```python
from build123d import *

# Parameters (mm, degrees)
SKETCH1_W           = 150
SKETCH1_H           = 60
BOSS_EXTRUDE1_DEPTH = 20
SKETCH2_W           = 22
SKETCH2_H           = 60
BOSS_EXTRUDE2_DEPTH = 10
SKETCH3_W           = 26.3
SKETCH3_H           = 26.3
CUT_EXTRUDE1_DEPTH  = 84.216584885
SKETCH4_R           = 2.2
CUT_EXTRUDE2_DEPTH  = 101.623058987
SKETCH5_R           = 2.8
CUT_EXTRUDE3_DEPTH  = 6
SKETCH6_R           = 4
CUT_EXTRUDE4_DEPTH  = 2


with BuildPart() as part:
    # Sketch1 → Boss-Extrude1 (new body)
    with BuildSketch(Plane(origin=(0, 0, 0), x_dir=(1, 0, 0), z_dir=(0, 1, 0))):
        Rectangle(SKETCH1_W, SKETCH1_H)
    extrude(amount=BOSS_EXTRUDE1_DEPTH)

    # Sketch2 → Boss-Extrude2 (add)
    with BuildSketch(Plane(origin=(0, 20, 0), x_dir=(1, 0, 0), z_dir=(0, 1, 0))):
        with Locations((-64, 0)):
            Rectangle(SKETCH2_W, SKETCH2_H)
    extrude(amount=BOSS_EXTRUDE2_DEPTH)

    # Sketch3 → Cut-Extrude1 (cut, through all)
    with BuildSketch(Plane(origin=(0, 20, 0), x_dir=(1, 0, 0), z_dir=(0, 1, 0))):
        with Locations((-22.5, 0)):
            Rectangle(SKETCH3_W, SKETCH3_H)
    extrude(amount=-CUT_EXTRUDE1_DEPTH, mode=Mode.SUBTRACT)

    # Sketch4 → Cut-Extrude2 (cut, through all)
    with BuildSketch(Plane.XY.offset(30)):
        with Locations((-22.5, 10)):
            Circle(SKETCH4_R)
    extrude(amount=-CUT_EXTRUDE2_DEPTH, mode=Mode.SUBTRACT)

    # Sketch5 → Cut-Extrude3 (cut)
    with BuildSketch(Plane.XY.offset(30)):
        with Locations((-22.5, 10)):
            Circle(SKETCH5_R)
    extrude(amount=-CUT_EXTRUDE3_DEPTH, mode=Mode.SUBTRACT)

    # Sketch6 → Cut-Extrude4 (cut)
    with BuildSketch(Plane(origin=(0, 0, 0), x_dir=(-1, 0, 0), z_dir=(0, -1, 0))):
        with Locations(Location((0, 0, 0), (0, 0, 90))):
            Circle(SKETCH6_R)
        with Locations(Location((-55, 0, 0), (0, 0, 90))):
            Circle(SKETCH6_R)
        with Locations(Location((55, 0, 0), (0, 0, 90))):
            Circle(SKETCH6_R)
    extrude(amount=-CUT_EXTRUDE4_DEPTH, mode=Mode.SUBTRACT)


solid = part.part
```
Check sheet for the modelled part. Datum: model origin and axes. Units: mm. A direction names the side the tool comes from. Round coordinates to 2 decimals unless told otherwise and drop trailing zeros. Loops run counter-clockwise (first coordinate to the right, second up) from the corner with the lowest first, then second, coordinate; pieces in that order, holes last. Notation, with made-up numbers: (-34, -37) - (-15, -37) arc R30 ccw to (-15, -9) - close; hole circle Ø11 at (79, 34). An arc over 180 degrees is marked (long way). Write item = value, one per line. Start each with the question number.
Q1. Section check A-A (x = -22.5). Record the boundary of the cut face in (y, z).
Q2. Section check D-D (y = 10). Record the boundary of the cut face in (x, z).
Q3. Section check C-C (z = 0). Record the boundary of the cut face in (x, y), plus the area to 3 significant figures.
Q4. Access from +Z, -Z, +X, -X, +Y, -Y to the whole of each face (thin tool, end or side, straight path). Record for faces 4 (the face through (-25.3, 10.1, 27)), 5 (the face through (-53, 25, 0)), 6 (the face through (55, 2, 0)), 7 (the face through (-22.7, 12.4, -13.15)), 8 (the face through (-20.4, 10.66, 18.65)).
Q5. Thickness scan on L1, parallel to X at y = 1.25, z = 0; L2, parallel to Y at x = 56, z = 25.5; L3, parallel to Z at x = -30.5, y = 1.75. Record the ranges inside material, lowest first.
Q6. Section check B-B (y = 17.25). Record the boundary of the cut face in (x, z).
Q7. Release check for a two-part mould opening along Y. For faces 1 (the face through (-64, 30, 0)), 2 (the face through (-1, 11, 30)), 3 (the face through (-21, 8, 24)) record: pulls with the +Y half, pulls with the -Y half, needs draft (parallel to the pull), parting line crosses it, or undercut.
Q8. Depth check by flat-ended pin: P1, Ø3.5, axis at x = -22.5, y = 10, coming from the -Z side; P2, Ø10.5, axis at x = 55, z = 0, coming from the +Y side; P3, Ø9, axis at x = -55.5, z = 1.5, coming from the -Y side; P4, Ø5, axis at y = 25.5, z = -5, coming from the +X side. Enter the tip coordinate at first touch or a pass-through.
Derived:
q1.outline = (0, -30) - (7.8, -30) - (7.8, -13.15) - (0, -13.15) - close; (0, 13.15) - (7.8, 13.15) - (7.8, 24) - (7.2, 24) - (7.2, 30) - (0, 30) - close; (12.2, -30) - (20, -30) - (20, -13.15) - (12.2, -13.15) - close; (12.2, 13.15) - (20, 13.15) - (20, 30) - (12.8, 30) - (12.8, 24) - (12.2, 24) - close
q2.outline = (-75, -30) - (-24.7, -30) - (-24.7, -13.15) - (-35.65, -13.15) - (-35.65, 13.15) - (-24.7, 13.15) - (-24.7, 24) - (-25.3, 24) - (-25.3, 30) - (-75, 30) - close; (-20.3, -30) - (75, -30) - (75, 30) - (-19.7, 30) - (-19.7, 24) - (-20.3, 24) - (-20.3, 13.15) - (-9.35, 13.15) - (-9.35, -13.15) - (-20.3, -13.15) - close
q3.outline = (-75, 0) - (-59, 0) - (-59, 2) - (-51, 2) - (-51, 0) - (-35.65, 0) - (-35.65, 20) - (-53, 20) - (-53, 30) - (-75, 30) - close; (-9.35, 0) - (-4, 0) - (-4, 2) - (4, 2) - (4, 0) - (51, 0) - (51, 2) - (59, 2) - (59, 0) - (75, 0) - (75, 20) - (-9.35, 20) - close
q3.area = 2,650 mm^2
q4.face_4 = +Z
q4.face_5 = +Z, -Z, +X, +Y
q4.face_6 = -Y
q4.face_7 = +Y, -Y
q4.face_8 = +Z, -Z
q5.L1 = -75 to -59, -51 to -35.65, -9.35 to -4, 4 to 51, 59 to 75
q5.L2 = 0 to 20
q5.L3 = -30 to -13.15, 13.15 to 30
q6.outline = (-75, -30) - (75, -30) - (75, 30) - (-75, 30) - close; hole (-35.65, -13.15) - (-9.35, -13.15) - (-9.35, 13.15) - (-35.65, 13.15) - close
q7.face_1 = pulls with the +Y half
q7.face_2 = needs draft
q7.face_3 = undercut
q8.P1 = through
q8.P2 = 20
q8.P3 = 0
q8.P4 = -53
